Verification items for the finished model (mm, model axes). Coordinates: 2 decimals unless noted, no trailing zeros. Order: outer loops, then holes, each group sorted by start corner. A loop starts at its lowest first (then second) coordinate and runs counter-clockwise, first axis right, second up. Notation, with made-up numbers: M 34,-36 L 86,-36 A28 cw 86,-16 Z; hole C 56,1 d5. An arc over 180 degrees is marked long. Return JSON: item names as keys, results as strings. Group by question number.
Q1. Section check C-C, the plane x = -44.45. Enter the section's corners in (y, z).
Q2. Section check B-B, the plane z = -38.1. Enter the section's corners in (x, y), then the cut area to 3 significant figures.
Q3. Go/stop test with a flat-tipped pin: pin 1 Ø8 at (x, z) = (-170, 77.5) entering from +Y. Record where the tip stops, or that it passes through.
Q4. Thickness scan on probe 1 along X at (y, z) = (-2.7, -114); probe 2 along Z at (x, y) = (209.55, -3.75); probe 3 along Z at (x, y) = (130, -0.5). Record the ranges inside material, lowest first.
Q5. Mould release check, pull along Z, two halves, no side actions. Record for faces 1 (the face through (-207.22, -2.35, -118.77)), 2 (the face through (-3, 0, 2)): pulls with the +Z half, pulls with the -Z half, needs draft (parallel to the pull), parting line crosses it, or undercut.
Q6. Section check D-D, the plane z = 38.1. Enter the section's corners in (x, y), then the cut area to 3 significant figures.
Q7. Section check A-A, the plane x = -133.5. Enter the section's corners in (y, z).
from build123d import *

# Parameters (mm, degrees)
F0_W     = 444.5
F0_H     = 254
F0_R     = 5.0419
F0_R_2   = 25.4
F1_DEPTH = 4.7625


with BuildPart() as f1:
    # F0 (on Front) → F1 (new body)
    with BuildSketch(Plane.XZ):
        Rectangle(F0_W, F0_H)
        with Locations((-209.55, -114.3)):
            Circle(F0_R, mode=Mode.SUBTRACT)
        with Locations((-209.55, -38.1)):
            Circle(F0_R, mode=Mode.SUBTRACT)
        Polygon((-143.424647, -63.5), (-138.387323, -54.7751), (-128.312677, -54.7751), (-123.275353, -63.5), (-128.312677, -72.2249), (-138.387323, -72.2249), align=None, mode=Mode.SUBTRACT)
        Polygon((-54.524647, -63.5), (-49.487323, -54.7751), (-39.412677, -54.7751), (-34.375353, -63.5), (-39.412677, -72.2249), (-49.487323, -72.2249), align=None, mode=Mode.SUBTRACT)
        with Locations((209.55, -114.3)):
            Circle(F0_R, mode=Mode.SUBTRACT)
        Polygon((34.375353, -63.5), (39.412677, -54.7751), (49.487323, -54.7751), (54.524647, -63.5), (49.487323, -72.2249), (39.412677, -72.2249), align=None, mode=Mode.SUBTRACT)
        Polygon((123.275353, -63.5), (128.312677, -54.7751), (138.387323, -54.7751), (143.424647, -63.5), (138.387323, -72.2249), (128.312677, -72.2249), align=None, mode=Mode.SUBTRACT)
        with Locations((209.55, -38.1)):
            Circle(F0_R, mode=Mode.SUBTRACT)
        Polygon((-143.424647, 0), (-138.387323, 8.7249), (-128.312677, 8.7249), (-123.275353, 0), (-128.312677, -8.7249), (-138.387323, -8.7249), align=None, mode=Mode.SUBTRACT)
        with Locations((-209.55, 38.1)):
            Circle(F0_R, mode=Mode.SUBTRACT)
        with Locations((-44.45, 31.75)):
            Circle(F0_R_2, mode=Mode.SUBTRACT)
        Polygon((-143.424647, 63.5), (-138.387323, 72.2249), (-128.312677, 72.2249), (-123.275353, 63.5), (-128.312677, 54.7751), (-138.387323, 54.7751), align=None, mode=Mode.SUBTRACT)
        with Locations((-209.55, 114.3)):
            Circle(F0_R, mode=Mode.SUBTRACT)
        Polygon((34.375353, 0), (39.412677, 8.7249), (49.487323, 8.7249), (54.524647, 0), (49.487323, -8.7249), (39.412677, -8.7249), align=None, mode=Mode.SUBTRACT)
        Polygon((123.275353, 0), (128.312677, 8.7249), (138.387323, 8.7249), (143.424647, 0), (138.387323, -8.7249), (128.312677, -8.7249), align=None, mode=Mode.SUBTRACT)
        with Locations((209.55, 38.1)):
            Circle(F0_R, mode=Mode.SUBTRACT)
        Polygon((34.375353, 63.5), (39.412677, 72.2249), (49.487323, 72.2249), (54.524647, 63.5), (49.487323, 54.7751), (39.412677, 54.7751), align=None, mode=Mode.SUBTRACT)
        Polygon((123.275353, 63.5), (128.312677, 72.2249), (138.387323, 72.2249), (143.424647, 63.5), (138.387323, 54.7751), (128.312677, 54.7751), align=None, mode=Mode.SUBTRACT)
        with Locations((209.55, 114.3)):
            Circle(F0_R, mode=Mode.SUBTRACT)
    extrude(amount=F1_DEPTH)


solid = f1.part
Numbers:
{
 "1": {"outline": "M -4.76,-127 L 0,-127 L 0,-72.22 L -4.76,-72.22 Z; M -4.76,-54.78 L 0,-54.78 L 0,6.35 L -4.76,6.35 Z; M -4.76,57.15 L 0,57.15 L 0,127 L -4.76,127 Z"},
 "2": {"outline": "M -222.25,-4.76 L -214.59,-4.76 L -214.59,0 L -222.25,0 Z; M -204.51,-4.76 L 204.51,-4.76 L 204.51,0 L -204.51,0 Z; M 214.59,-4.76 L 222.25,-4.76 L 222.25,0 L 214.59,0 Z", "area": "2,020 mm2"},
 "3": {"pin 1": "stops at y = 0"},
 "4": {"probe 1": "x = -222.25 to -214.58, -204.52 to 204.52, 214.58 to 222.25", "probe 2": "z = -127 to -119.34, -109.26 to -43.14, -33.06 to 33.06, 43.14 to 109.26, 119.34 to 127", "probe 3": "z = -127 to -72.22, -54.78 to -8.72, 8.72 to 54.78, 72.22 to 127"},
 "5": {"face 1": "undercut", "face 2": "needs draft"},
 "6": {"outline": "M -222.25,-4.76 L -214.59,-4.76 L -214.59,0 L -222.25,0 Z; M -204.51,-4.76 L -69.04,-4.76 L -69.04,0 L -204.51,0 Z; M -19.86,-4.76 L 204.51,-4.76 L 204.51,0 L -19.86,0 Z; M 214.59,-4.76 L 222.25,-4.76 L 222.25,0 L 214.59,0 Z", "area": "1,790 mm2"},
 "7": {"outline": "M -4.76,-127 L 0,-127 L 0,-72.22 L -4.76,-72.22 Z; M -4.76,-54.78 L 0,-54.78 L 0,-8.72 L -4.76,-8.72 Z; M -4.76,8.72 L 0,8.72 L 0,54.78 L -4.76,54.78 Z; M -4.76,72.22 L 0,72.22 L 0,127 L -4.76,127 Z"}
}
